Work out the finished part from the listing and answer in its coordinate system (mm). Face numbers are marked on the shaded views. A direction names the side the tool comes from. Round coordinates to 2 decimals unless told otherwise and drop trailing zeros. Loops run counter-clockwise (first coordinate to the right, second up) from the corner with the lowest first, then second, coordinate; pieces in that order, holes last.
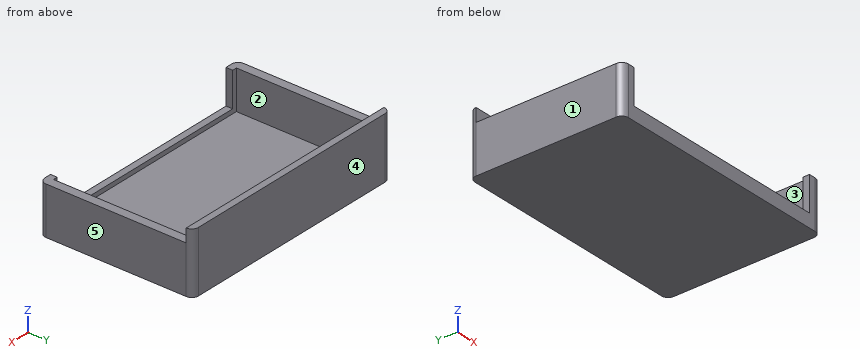
```python
from build123d import *

# Parameters (mm, degrees)
F0_W     = 107
F0_H     = 6
F1_DEPTH = 69
F3_DEPTH = 15.5
F4_W     = 2
F4_H     = 63
F4_W_2   = 95
F5_DEPTH = 17.5
F6_DEPTH = 6
F7_R     = 2.99999


# Not quite as in the source:
# - a fillet or chamfer is up to 0.001 mm smaller than in the source, because OpenCascade refuses the exact size


with BuildPart() as f1:
    # F0 (on Front) → F1 (new body)
    with BuildSketch(Plane.XZ):
        with Locations((0, 3)):
            Rectangle(F0_W, F0_H)
    extrude(amount=F1_DEPTH)

    # F2 (on face) → F3 (join)
    with BuildSketch(Plane.XY.offset(6)):
        Polygon((53.5, -3), (53.5, 0), (47.5, 0), (-47.5, 0), (-53.5, 0), (-53.5, -3), (-53.5, -69), (-47.5, -69), (-47.5, -3), (47.5, -3), (47.5, -69), (53.5, -69), align=None)
    extrude(amount=F3_DEPTH)

    # F4 (on face) → F5 (cut)
    with BuildSketch(Plane.XY.offset(21.5)):
        with Locations((-48.5, -34.5)):
            Rectangle(F4_W, F4_H)
        with Locations((0, -34.5)):
            Rectangle(F4_W_2, F4_H)
        with Locations((48.5, -34.5)):
            Rectangle(F4_W, F4_H)
    extrude(amount=-F5_DEPTH, mode=Mode.SUBTRACT)

    # F4 (on face) → F6 (join)
    with BuildSketch(Plane.XY.offset(21.5)):
        Polygon((-53.5, -3), (-49.5, -3), (-47.5, -3), (47.5, -3), (49.5, -3), (53.5, -3), (53.5, 0), (-53.5, 0), align=None)
    extrude(amount=F6_DEPTH)

    # F7 (radius 3 in the source; OpenCascade refuses exactly that, so slightly less here)
    f7_edges = [f1.edges().sort_by_distance(p)[0] for p in [
        (-53.5, -69, 10.75),
        (53.5, -69, 10.75),
        (53.5, 0, 13.75),
        (-53.5, 0, 13.75),
    ]]
    fillet(f7_edges, radius=F7_R)


solid = f1.part
```
1. Determine the mould class of the marked faces 3, 4 and 5 for opening direction Y: +Y half, -Y half, draft (parallel to the pull), parting line (faces both ways), or undercut.
Answer key:
face 3: undercut
face 4: +Y half
face 5: draft
2. Find section B-B (x = -41.5). Write down the section's boundary in (y, z).
Answer key:
outline: (-69, 0) - (0, 0) - (0, 27.5) - (-3, 27.5) - (-3, 4) - (-66, 4) - (-66, 6) - (-69, 6) - close
3. Consider probe 1 along X at (y, z) = (-21, 8); probe 2 along Y at (x, z) = (-28, 21.75); probe 3 along Z at (x, y) = (-35, -32.5). Determine where each line is inside the solid, lowest interval first.
Answer key:
probe 1: x = -53.5 to -49.5, 49.5 to 53.5
probe 2: y = -3 to 0
probe 3: z = 0 to 4
4. Find section D-D (z = 13.75). Write down the section's boundary in (x, y), then the cut area to 3 significant figures.
Answer key:
outline: (-53.5, -66) arc R3 ccw to (-50.5, -69) - (-47.5, -69) - (-47.5, -66) - (-49.5, -66) - (-49.5, -3) - (49.5, -3) - (49.5, -66) - (47.5, -66) - (47.5, -69) - (50.5, -69) arc R3 ccw to (53.5, -66) - (53.5, -3) arc R3 ccw to (50.5, 0) - (-50.5, 0) arc R3 ccw to (-53.5, -3) - close
area: 853 mm2
5. Given pin 1 (1.5 mm diameter, centred on y = -68, z = 16.5, fed in from +X); pin 2 (1.5 mm diameter, centred on x = 28.5, z = 22.5, fed in from -Y); pin 3 (1.8 mm diameter, centred on x = -51, y = -47, fed in from +Z), each flat-ended and moving along its own axis, determine where each tip first touches the part or whether it passes through.
Answer key:
pin 1: stops at x = 53.23
pin 2: stops at y = -3
pin 3: stops at z = 21.5
6. Find section A-A (y = -39). Write down the section's boundary in (x, z).
Answer key:
outline: (-53.5, 0) - (53.5, 0) - (53.5, 21.5) - (49.5, 21.5) - (49.5, 4) - (-49.5, 4) - (-49.5, 21.5) - (-53.5, 21.5) - close
7. Which of the six approach directions +Z, -Z, +X, -X, +Y, -Y give full straight-line access (tool end or side, diameter ignored) to the marked faces 1 and 2?
Answer key:
face 1: +Z, -Z, -X, +Y, -Y
face 2: +Z
